from build123d import *

# Parameters (mm, degrees)
MAGNET_SLOT_DEPTH   = 2.6
MAGNET_TOPPER_DEPTH = 0.6
BOTTOM_START        = 0.4
BOTTOM_DEPTH        = 0.4
CUT_EXTRUDE1_REACH  = 31.916
FILLET1_R           = 1
BOSS_EXTRUDE1_DEPTH = 3.9
CHAMFER1_SIZE       = 0.8
CHAMFER2_SIZE       = 1
CIRPATTERN1_COUNT   = 4


with BuildPart() as part:
    # Sketch1 → Magnet Slot (new body)
    with BuildSketch(Plane.XY):
        with BuildLine():
            Line((-21, 0), (-18.7, 0))
            Line((-18.7, 0), (-18.7, 8.45))
            Line((-18.7, 8.45), (-13.423469406, 8.45))
            ThreePointArc((-13.423469406, 8.45), (-13.215070921, 8.56190557), (-13.193240046, 8.797439428))
            Line((-13.193240046, 8.797439428), (-13.513172798, 9.553374824))
            ThreePointArc((-13.513172798, 9.553374824), (-14.998097039, 14.998097039), (-9.553374824, 13.513172798))
            Line((-9.553374824, 13.513172798), (-8.797439428, 13.193240046))
            ThreePointArc((-8.797439428, 13.193240046), (-8.56190557, 13.215070921), (-8.45, 13.423469406))
            Line((-8.45, 13.423469406), (-8.45, 18.7))
            Line((-8.45, 18.7), (0, 18.7))
            Line((0, 18.7), (0, 21))
            Line((0, 21), (-21, 21))
            Line((-21, 21), (-21, 0))
        make_face()
    extrude(amount=MAGNET_SLOT_DEPTH)

    # Sketch2 → Magnet Topper (add)
    with BuildSketch(Plane.XY.offset(2.6)):
        with BuildLine():
            Line((-12.7, 8.45), (-18.7, 8.45))
            Line((-18.7, 8.45), (-18.7, 0))
            Line((-18.7, 0), (-21, 0))
            Line((-21, 0), (-21, 21))
            Line((-21, 21), (0, 21))
            Line((0, 21), (0, 18.7))
            Line((0, 18.7), (-8.45, 18.7))
            Line((-8.45, 18.7), (-8.45, 12.7))
            ThreePointArc((-8.45, 12.7), (-9.69479618, 9.69479618), (-12.7, 8.45))
        make_face()
    extrude(amount=MAGNET_TOPPER_DEPTH)

    # Sketch3 → Bottom (add)
    with BuildSketch(Plane(origin=(0, 0, 0), x_dir=(-1, 0, 0), z_dir=(0, 0, -1)).offset(BOTTOM_START)):
        with BuildLine():
            Line((18.7, 8.45), (18.7, 0))
            Line((18.7, 0), (21, 0))
            Line((21, 0), (21, 21))
            Line((21, 21), (0, 21))
            Line((0, 21), (0, 18.7))
            Line((0, 18.7), (8.45, 18.7))
            Line((8.45, 18.7), (8.45, 12.7))
            ThreePointArc((8.45, 12.7), (9.69479618, 9.69479618), (12.7, 8.45))
            Line((12.7, 8.45), (18.7, 8.45))
        make_face()
    extrude(amount=-BOTTOM_DEPTH)

    # Cut-Extrude1: up to this face of the body (flat: up to its plane)
    cut_extrude1_end = Plane(part.part.faces().sort_by_distance((-12.297393308, 12.297393308, 2.6))[0])
    # Sketch4 → Cut-Extrude1 (cut, up to the picked face)
    with BuildSketch(Plane(origin=(0, 0, -0.4), x_dir=(-1, 0, 0), z_dir=(0, 0, -1)), mode=Mode.PRIVATE) as cut_extrude1_sk1:
        with BuildLine():
            Line((11.992893219, 13.407106781), (15.528427125, 16.942640687))
            ThreePointArc((15.528427125, 16.942640687), (16.942640687, 16.942640687), (16.942640687, 15.528427125))
            Line((16.942640687, 15.528427125), (13.407106781, 11.992893219))
            ThreePointArc((13.407106781, 11.992893219), (11.992893219, 11.992893219), (11.992893219, 13.407106781))
        make_face()
    cut_extrude1_tool1 = split(extrude(cut_extrude1_sk1.sketch, amount=-CUT_EXTRUDE1_REACH, mode=Mode.PRIVATE), bisect_by=cut_extrude1_end, keep=Keep.BOTH, mode=Mode.PRIVATE)
    add(cut_extrude1_tool1.solids().sort_by(Axis((-14.467767, 14.467767, -0.4), (0, 0, 1)))[0], mode=Mode.SUBTRACT)

    # Fillet1
    fillet1_edges = [part.edges().sort_by_distance(p)[0] for p in [
        (-8.45, 18.7, 1.4),
        (-18.7, 8.45, 1.4),
    ]]
    fillet(fillet1_edges, radius=FILLET1_R)

    # Sketch5 → Boss-Extrude1 (add)
    with BuildSketch(Plane.XY.offset(3.2)):
        with BuildLine():
            Line((0, 21), (-17.25, 21))
            Line((-17.25, 21), (-21, 21))
            Line((-21, 21), (-21, 17.25))
            Line((-21, 17.25), (-21, 0))
            Line((-21, 0), (-19.25, 0))
            Line((-19.25, 0), (-19.25, 17))
            ThreePointArc((-19.25, 17), (-18.590990258, 18.590990258), (-17, 19.25))
            Line((-17, 19.25), (0, 19.25))
            Line((0, 19.25), (0, 21))
        make_face()
    extrude(amount=BOSS_EXTRUDE1_DEPTH)

    # Chamfer1
    chamfer1_edges = [part.edges().sort_by_distance(p)[0] for p in [
        (-19.25, 8.5, 3.2),
        (-18.590990258, 18.590990258, 3.2),
        (-8.5, 19.25, 3.2),
    ]]
    chamfer(chamfer1_edges, length=CHAMFER1_SIZE)

    # Chamfer2
    chamfer2_edges = [part.edges().sort_by_distance(p)[0] for p in [
        (-19.25, 8.5, 7.1),
        (-18.590990258, 18.590990258, 7.1),
        (-8.5, 19.25, 7.1),
    ]]
    chamfer(chamfer2_edges, length=CHAMFER2_SIZE)


with BuildPart() as cirpattern1_1:
    # CirPattern1: pattern copy
    add(part.part.rotate(Axis((0, 0, 0), (0, 0, 1)), 1 * 360 / CIRPATTERN1_COUNT))


with BuildPart() as cirpattern1_2:
    # CirPattern1: pattern copy
    add(part.part.rotate(Axis((0, 0, 0), (0, 0, 1)), 2 * 360 / CIRPATTERN1_COUNT))


with BuildPart() as cirpattern1_3:
    # CirPattern1: pattern copy
    add(part.part.rotate(Axis((0, 0, 0), (0, 0, 1)), 3 * 360 / CIRPATTERN1_COUNT))


with BuildPart() as part_1:
    add(part.part)

    # Combine1: union CirPattern1_3, CirPattern1_1, CirPattern1_2
    add(cirpattern1_3.part)
    add(cirpattern1_1.part)
    add(cirpattern1_2.part)


solid = part_1.part
Work out the finished part from the listing and answer in its coordinate system (mm). A direction names the side the tool comes from. Give positions to 0.01 mm unless a question says otherwise; leave off trailing zeros. Loops run counter-clockwise (first coordinate to the right, second up) from the corner with the lowest first, then second, coordinate; pieces in that order, holes last. Notation, with made-up numbers: (56, 53) -> (75, 53) arc R8 ccw to (75, 65) -> close; hole circle Ø2 at (85.25, 2). An arc over 180 degrees is marked (long way). Use a Markdown table: item, result. Add a question column.
1. Section A-A on x = 15 is taken. Determine the outline of the cut face in (y, z).
2. Find the intervals of material crossed by probe 1 along X at (y, z) = (-3, 5.5); probe 2 along X at (y, z) = (7, 1.5), in increasing order.
3. For faces 1 (the cylindrical face through (9.73, 9.66, -0.2)), 2 (the conical face through (18.891, -18.85, 6.496)), 3 (the flat face through (11, 12, 0)), 4 (the cylindrical face through (-16.958, -16.927, 1.079)), determine the directions among +Z, -Z, +X, -X, +Y, -Y from which every point of the face is accessible in a straight line to the end or side of a thin tool.
4. Section C-C on x = 3 is taken. Determine the outline of the cut face in (y, z).
5. Determine the mould class of faces 5 (the flat face through (21, 0, 3)), 6 (the cylindrical face through (15.647, -11.33, 1.282)), 7 (the cylindrical face through (-11.33, -15.647, 1.282)) for opening direction Y: released by +Y, released by -Y, zero draft, split by the parting line, or undercut.
6. Flat-ended cylindrical pins translate along their axes: pin 1 Ø5 at (x, y) = (-12, 16) entering from +Z; pin 2 Ø2 at (x, y) = (6, -15) entering from +Z. Find the tip coordinate at first contact, or state that the pin passes through.
Results below:
| question | item | result |
|---|---|---|
| 1 | outline | (-21, -0.4) -> (-16.41, -0.4) -> (-16.41, 2.6) -> (-10.4, 2.6) -> (-10.4, 0) -> (-13.59, 0) -> (-13.59, -0.4) -> (-8.45, -0.4) -> (-8.45, 3.2) -> (-18.45, 3.2) -> (-19.25, 4) -> (-19.25, 6.1) -> (-20.25, 7.1) -> (-21, 7.1) -> close; (8.45, -0.4) -> (13.59, -0.4) -> (13.59, 0) -> (10.4, 0) -> (10.4, 2.6) -> (16.41, 2.6) -> (16.41, -0.4) -> (21, -0.4) -> (21, 7.1) -> (20.25, 7.1) -> (19.25, 6.1) -> (19.25, 4) -> (18.45, 3.2) -> (8.45, 3.2) -> close |
| 2 | probe 1 | x = -21 to -19.25, 19.25 to 21 |
| 2 | probe 2 | x = -21 to -18.7, 18.7 to 21 |
| 3 | face 1 | +Z, -Z |
| 3 | face 2 | +Z |
| 3 | face 3 | none |
| 3 | face 4 | -Z |
| 4 | outline | (-21, -0.4) -> (-18.7, -0.4) -> (-18.7, 3.45) -> (-19.25, 4) -> (-19.25, 6.1) -> (-20.25, 7.1) -> (-21, 7.1) -> close; (18.7, -0.4) -> (21, -0.4) -> (21, 7.1) -> (20.25, 7.1) -> (19.25, 6.1) -> (19.25, 4) -> (18.7, 3.45) -> close |
| 5 | face 5 | zero draft |
| 5 | face 6 | undercut |
| 5 | face 7 | undercut |
| 6 | pin 1 | stops at z = 3.25 |
| 6 | pin 2 | passes through |
